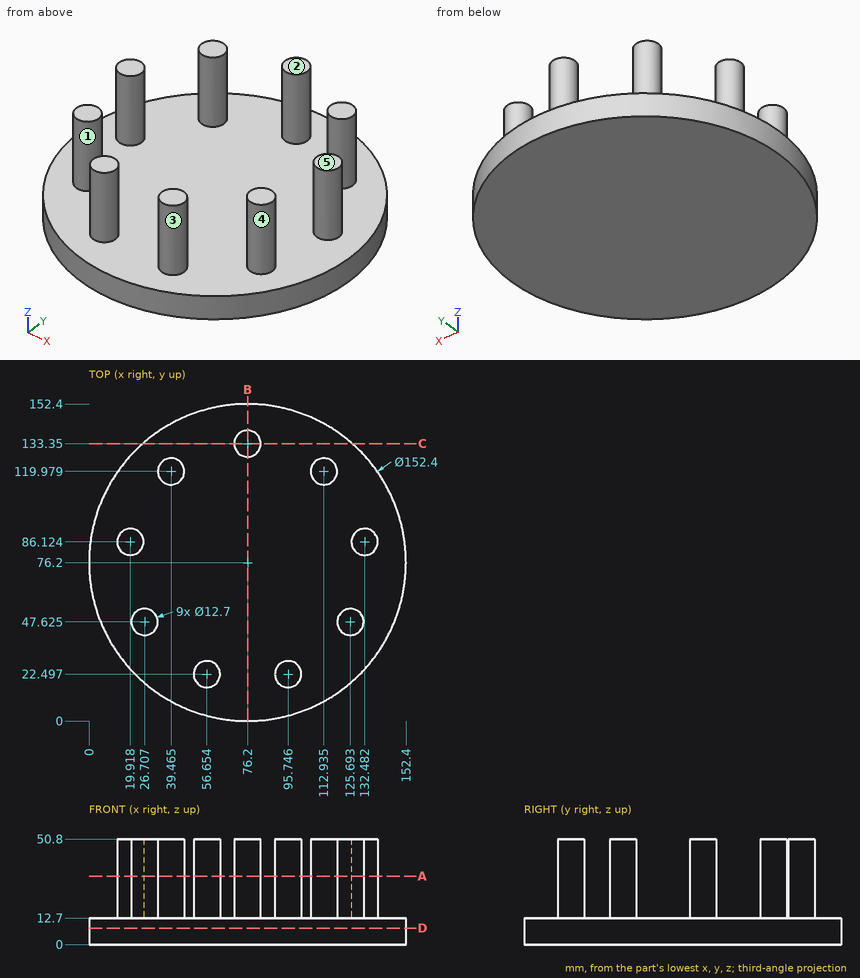
Design review of the part shown in the three views and the two pictorial views. Dimensions are in mm from the part's minimum x, y and z. A direction names the side the tool comes from. Coordinates: 2 decimals unless noted, no trailing zeros. Write each loop counter-clockwise with the first axis right and the second up, starting at its lowest first coordinate (ties: lowest second). Pieces come first, ordered by that corner, then holes.
1) Clearance check with flat-ended pins moving along their axes: pin 1 Ø12 at (y, z) = (89.5, 39.5) entering from -X; pin 2 Ø2 at (y, z) = (126, 16) entering from +X (1 decimal); pin 3 Ø4 at (y, z) = (84, 25.5) entering from +X. State where each tip first meets the part, or that it passes through.
2) The part is to be moulded in two halves that separate along Y. For the marked faces 1, 2 and 3, say which applies: pulls with the +Y half, pulls with the -Y half, needs draft (parallel to the pull), parting line crosses it, or undercut.
3) We need section C-C on y = 133.35. State the section outline as (x, z) points, then the cut area to 3 significant figures.
4) We need section D-D on z = 8. State the section outline as (x, y) points.
5) Machinability: for the marked faces 4 and 5, which of the approach directions +Z, -Z, +X, -X, +Y, -Y give a long, thin tool a straight path to every point of the face, cutting with its end or side? Answer none if there is none.
6) To check wall thickness, follow probe 1 along X at (y, z) = (116.5, 42) (1 decimal); probe 2 along X at (y, z) = (17, 38) (1 decimal); probe 3 along Z at (x, y) = (141.5, 109). State the ranges of each line that lie inside material, in increasing order.
7) We need section A-A on z = 33. Count the separate pieces of the cut face and the enclosed holes in it, then the cut area to 3 significant figures.
8) We need section B-B on x = 76.2. State the section outline as (y, z) points.
Answer list:
1. pin 1: stops at x = 13.57
1. pin 2: stops at x = 116.8
1. pin 3: stops at x = 138.83
2. face 1: undercut
2. face 2: needs draft
2. face 3: parting line crosses it
3. outline: (25.8, 0) - (126.6, 0) - (126.6, 12.7) - (82.55, 12.7) - (82.55, 50.8) - (69.85, 50.8) - (69.85, 12.7) - (25.8, 12.7) - close
3. area: 1,760 mm2
4. outline: circle Ø152.4 at (76.2, 76.2)
5. face 4: +Z
5. face 5: +Z, +X, -X, +Y, -Y
6. probe 1: x = 34.2 to 44.8, 107.6 to 118.2
6. probe 2: x = 53.5 to 59.8, 92.6 to 98.9
6. probe 3: z = 0 to 12.7
7. separate pieces: 9
7. enclosed holes: 0
7. area: 1,140 mm2
8. outline: (0, 0) - (152.4, 0) - (152.4, 12.7) - (139.7, 12.7) - (139.7, 50.8) - (127, 50.8) - (127, 12.7) - (0, 12.7) - close
